Autodesk Inventor part; units mm, degrees
ref_plane "YZ Plane" through (0, 0, 0) normal (1, 0, 0) x (0, 1, 0)
ref_plane "XZ Plane" through (0, 0, 0) normal (0, 1, 0) x (-1, 0, 0)
ref_plane "XY Plane" through (0, 0, 0) normal (0, 0, 1) x (1, 0, 0)
sketch "Sketch1" plane through (0, 0, 0) normal (0, 0, 1) x (1, 0, 0)
  line L0 (0, 0) -> (25.4, 0)
  line L1 (25.4, 0) -> (25.4, 50.8)
  line L2 (25.4, 50.8) -> (0, 50.8)
  line L3 (0, 50.8) -> (0, 0)
  dimension "d0" = 25.4
  dimension "d1" = 50.8
extrude "Extrusion1" add sketch "Sketch1" along normal blind 127
shell "Shell1" thickness 3.175 removed faces 2 at (8.4667, 33.8667, 0) at (8.4667, 33.8667, 127)
sketch "Sketch3" plane through (0, 50.8, 0) normal (0, 1, 0) x (1, 0, 0)
  line L0 (0, -127) -> (25.4, -127)
  line L1 (25.4, 0) -> (25.4, -127)
  line L2 (25.4, 0) -> (0, 0)
  line L3 (0, 0) -> (0, -127)
  circle A0 centre (12.7, -9.525) radius 3.175
  circle A1 centre (12.7, -117.475) radius 3.175
  dimension "d10" = 6.35
  dimension "d11" = 12.7
  dimension "d12" = 9.525
  dimension "d13" = 12.7
  dimension "d14" = 9.525
sketch "Sketch2" plane through (25.4, 0, 0) normal (1, 0, 0) x (0, 0, -1)
  line L0 (-127, 50.8) -> (-127, 0)
  line L1 (0, 0) -> (-127, 0)
  line L2 (0, 0) -> (0, 50.8)
  line L3 (0, 50.8) -> (-127, 50.8)
  line L4 (-104.775, 50.8) -> (-22.225, 50.8)
  line L5 (-22.225, 50.8) -> (-22.225, 6.35)
  line L6 (-22.225, 6.35) -> (-104.775, 6.35)
  line L7 (-104.775, 6.35) -> (-104.775, 50.8)
  line L8 (-22.225, 35.4291) -> (0, 35.4291) construction
  line L9 (-104.775, 35.4291) -> (-127, 35.4291) construction
  dimension "d5" = 6.35
  dimension "d19" = 82.55
extrude "Extrusion3" cut sketch "Sketch3" against normal up to next contours A0 | A1
extrude "Extrusion4" cut sketch "Sketch2" against normal through all contours L3 L5 L6 L7
properties part number "Frame_BatteryMount" material "Aluminum-6061"
For this review, take the finished solid that the model builds, in its own axes (mm). A direction names the side the tool comes from. Round coordinates to 2 decimals unless told otherwise and drop trailing zeros. Order: outer loops, then holes, each group sorted by start corner. A loop starts at its lowest first (then second) coordinate and runs counter-clockwise, first axis right, second up.
Q1. Wall thickness on line 1 (Z direction, x = 12.7, y = 48.45) (3 decimals); line 2 (X direction, y = 9.5, z = 7) (3 decimals); line 3 (Y direction, x = 20.25, z = 7) (3 decimals): over which ranges is each line inside the solid? List them lowest first.
Findings below:
line 1: z = 0 to 6.35, 12.7 to 22.225, 104.775 to 114.3, 120.65 to 127
line 2: x = 0 to 3.175, 22.225 to 25.4
line 3: y = 0 to 3.175, 47.625 to 50.8
Q2. We need section D-D, the plane z = 68. Give the boundary of the cut face in (x, y) (3 decimals).
Findings below:
outline: (0, 0) - (25.4, 0) - (25.4, 6.35) - (22.225, 6.35) - (22.225, 3.175) - (3.175, 3.175) - (3.175, 6.35) - (0, 6.35) - close
Q3. Machinability: for faces 1 (the cylindrical face through (12.012, 49.235, 120.574)), 2 (the flat face through (2, 33, 104.775)), 3 (the flat face through (22.225, 5, 63)), which of the approach directions +Z, -Z, +X, -X, +Y, -Y give a long, thin tool a straight path to every point of the face, cutting with its end or side? Answer none if there is none.
Findings below:
face 1: +Y
face 2: +X, -X, +Y
face 3: +Z, -Z
Q4. We need section A-A, the plane y = 21.5. Give the boundary of the cut face in (x, z) (3 decimals).
Findings below:
outline: (0, 0) - (3.175, 0) - (3.175, 22.225) - (0, 22.225) - close; (0, 104.775) - (3.175, 104.775) - (3.175, 127) - (0, 127) - close; (22.225, 0) - (25.4, 0) - (25.4, 22.225) - (22.225, 22.225) - close; (22.225, 104.775) - (25.4, 104.775) - (25.4, 127) - (22.225, 127) - close
Q5. Mouldability with a two-part tool opening along X and no side actions: class faces 4 (the flat face through (0, 3, 63)), 5 (the cylindrical face through (10.18, 49.235, 11.457)), 6 (the flat face through (25.4, 2, 63)), 7 (the flat face through (13, 50.8, 113)) as pulls with the +X half, pulls with the -X half, needs draft (parallel to the pull), parting line crosses it, or undercut.
Findings below:
face 4: pulls with the -X half
face 5: undercut
face 6: pulls with the +X half
face 7: needs draft
Q6. We need section B-B, the plane x = 12.7. Give the boundary of the cut face in (y, z) (3 decimals), plus the area to 3 significant figures.
Findings below:
outline: (0, 0) - (3.175, 0) - (3.175, 127) - (0, 127) - close; (47.625, 0) - (50.8, 0) - (50.8, 6.35) - (47.625, 6.35) - close; (47.625, 12.7) - (50.8, 12.7) - (50.8, 22.225) - (47.625, 22.225) - close; (47.625, 104.775) - (50.8, 104.775) - (50.8, 114.3) - (47.625, 114.3) - close; (47.625, 120.65) - (50.8, 120.65) - (50.8, 127) - (47.625, 127) - close
area: 504 mm2
Q7. We need section C-C, the plane x = 6.25. Give the boundary of the cut face in (y, z) (3 decimals).
Findings below:
outline: (0, 0) - (3.175, 0) - (3.175, 127) - (0, 127) - close; (47.625, 0) - (50.8, 0) - (50.8, 22.225) - (47.625, 22.225) - close; (47.625, 104.775) - (50.8, 104.775) - (50.8, 127) - (47.625, 127) - close
Q8. Insertion check: P1, Ø3.5, axis at x = 24.5, z = 54.5, coming from the +Y side; P2, Ø5.5, axis at x = 10, z = 77, coming from the +Y side (3 decimals); P3, Ø3, axis at y = 8.5, z = 63, coming from the +X side. Each pin has a flat end and moves straight along its axis. Give the tip position at first contact, or say it passes through.
Findings below:
P1: stops at y = 6.35
P2: stops at y = 3.175
P3: passes through
